Verification items for this drawing (mm, ordinates from the low corner). Coordinates: 2 decimals unless noted, no trailing zeros. Write each loop counter-clockwise with the first axis right and the second up, starting at its lowest first coordinate (ties: lowest second). Pieces come first, ordered by that corner, then holes.
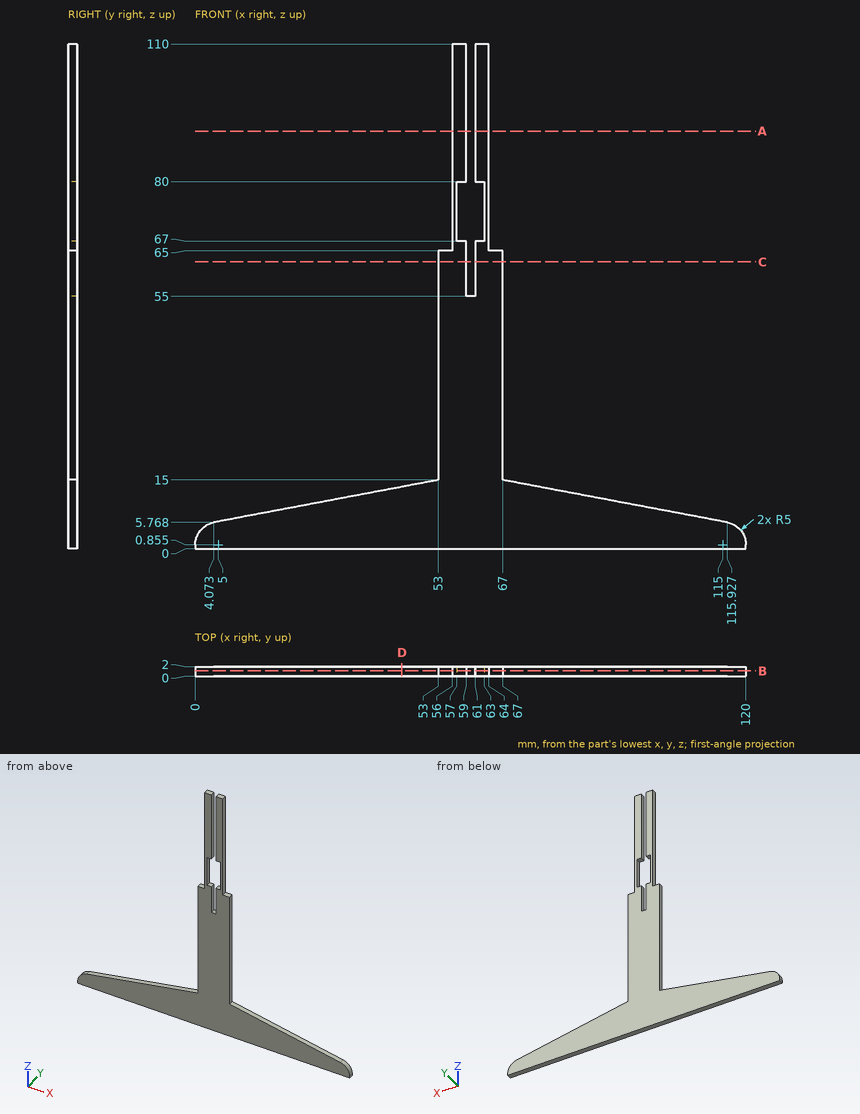
1. Sectioned sample at C-C, the plane z = 62.5. Record the boundary of the cut face in (x, y), and give its area (3 significant figures).
Computed values:
outline: (53, 0) - (59, 0) - (59, 2) - (53, 2) - close; (61, 0) - (67, 0) - (67, 2) - (61, 2) - close
area: 24.0 mm2
2. Sectioned sample at D-D, the plane x = 45. Record the boundary of the cut face in (y, z).
Computed values:
outline: (0, 0) - (2, 0) - (2, 13.49) - (0, 13.49) - close
3. Gauge pin test, flat ends, axial feed: pin 1 Ø0.6 at (y, z) = (1, 61) entering from +X; pin 2 Ø1 at (y, z) = (0.5, 71.5) entering from +X; pin 3 Ø1 at (y, z) = (1.5, 63) entering from -X. Record the tip position at first contact, or that the pin passes through.
Computed values:
pin 1: stops at x = 67
pin 2: stops at x = 64
pin 3: stops at x = 53
4. Sectioned sample at B-B, the plane y = 1.1. Record the boundary of the cut face in (x, z) (1 decimal).
Computed values:
outline: (0, 0) - (120, 0) - (120, 0.9) arc R5 ccw to (115.9, 5.8) - (67, 15) - (67, 65) - (64, 65) - (64, 110) - (61, 110) - (61, 80) - (63, 80) - (63, 67) - (61, 67) - (61, 55) - (59, 55) - (59, 67) - (57, 67) - (57, 80) - (59, 80) - (59, 110) - (56, 110) - (56, 65) - (53, 65) - (53, 15) - (4.1, 5.8) arc R5 ccw to (0, 0.9) - close
5. Sectioned sample at A-A, the plane z = 91. Record the boundary of the cut face in (x, y), and give its area (3 significant figures).
Computed values:
outline: (56, 0) - (59, 0) - (59, 2) - (56, 2) - close; (61, 0) - (64, 0) - (64, 2) - (61, 2) - close
area: 12.0 mm2
6. Thickness scan on line 1 along X through (y, z) = (1.5, 68); line 2 along X through (y, z) = (0.5, 94); line 3 along X through (y, z) = (1.15, 44.5). Record the ranges inside material, lowest first.
Computed values:
line 1: x = 56 to 57, 63 to 64
line 2: x = 56 to 59, 61 to 64
line 3: x = 53 to 67
